Input: part model. Units: mm. Frame: model coordinates. Face numbers are marked on the shaded views. A direction names the side the tool comes from. Coordinates: 2 decimals unless noted, no trailing zeros. Loops run counter-clockwise (first coordinate to the right, second up) from the corner with the lowest first, then second, coordinate; pieces in that order, holes last.
Item 1: Ray query, line 1 along Y through (x, z) = (0, 25); line 2 along Y through (x, z) = (0, 6.5); line 3 along Z through (x, y) = (-11, -6). Return the intervals inside material, ascending.
Item 2: Reachability of the marked faces 1, 2 and 3 from +Z, -Z, +X, -X, +Y, -Y: full face, straight path, thin tool, end or side. Return the list, or none.
Item 3: Section A-A on x = 0. Return loops of the section in (y, z), and give its area (3 significant figures).
Item 4: Section D-D on z = 20. Return loops of the section in (x, y), and give its area (3 significant figures).
Item 5: Pull-direction query (X, two-part tool) for the marked faces 4, 5 and 6; classes: released by +X, released by -X, zero draft, split by the parting line, or undercut.
Item 6: Section B-B on z = 7. Return loops of the section in (x, y).
Item 7: Section C-C on y = -21.5. Return loops of the section in (x, z).
Item 8: Contact query for flat-ended pins moving along their axis: P1, Ø4, axis at x = 28, z = 24, coming from the -Y side; P2, Ø1, axis at y = 32.5, z = 29.5, coming from the +X side; P3, Ø5.5, axis at x = 23.5, z = 5, coming from the -Y side; P4, Ø9, axis at x = 0, y = 0, coming from the +Z side. Output: stop coordinate, or through.
```python
from build123d import *

# Parameters (mm, degrees)
F0_R     = 39.624
F0_R_2   = 5.500002
F1_DEPTH = 12.7
F2_R     = 69.469
F2_R_2   = 39.624
F3_DEPTH = 21.7805
F5_DEPTH = 45.212


with BuildPart() as f1:
    # F0 (on Top) → F1 (new body)
    with BuildSketch(Plane.XY):
        Circle(F0_R)
        Circle(F0_R_2, mode=Mode.SUBTRACT)
    extrude(amount=F1_DEPTH)

    # F2 (on face) → F3 (join, symmetric)
    with BuildSketch(Plane.XY.offset(12.7)):
        Circle(F2_R)
        Circle(F2_R_2, mode=Mode.SUBTRACT)
    extrude(amount=F3_DEPTH, both=True)

    # F4 (on face) → F5 (cut)
    with BuildSketch(Plane.XY.offset(12.7)):
        Polygon((21.139988, -4.44315), (26.270496, -4.44315), (28.83575, 0), (26.270496, 4.44315), (21.139988, 4.44315), (18.574734, 0), align=None)
    extrude(amount=-F5_DEPTH, mode=Mode.SUBTRACT)


solid = f1.part
```
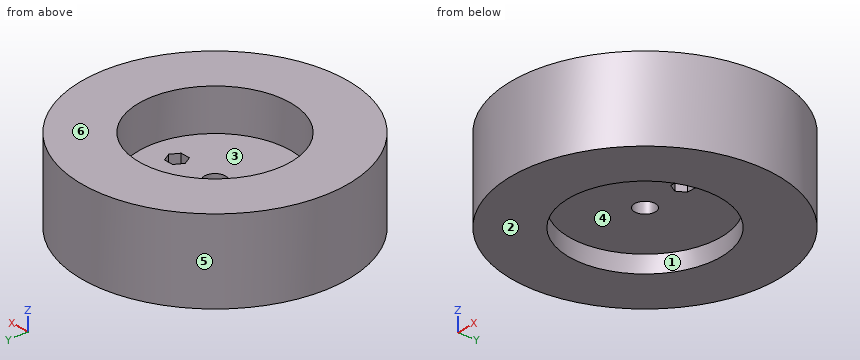
Results found:
1. line 1: y = -69.47 to -39.62, 39.62 to 69.47
1. line 2: y = -69.47 to -5.5, 5.5 to 69.47
1. line 3: z = 0 to 12.7
2. face 1: -Z
2. face 2: -Z, +X, -X, +Y, -Y
2. face 3: +Z
3. outline: (-69.47, -9.08) - (-39.62, -9.08) - (-39.62, 0) - (-5.5, 0) - (-5.5, 12.7) - (-39.62, 12.7) - (-39.62, 34.48) - (-69.47, 34.48) - close; (5.5, 0) - (39.62, 0) - (39.62, -9.08) - (69.47, -9.08) - (69.47, 34.48) - (39.62, 34.48) - (39.62, 12.7) - (5.5, 12.7) - close
3. area: 3,470 mm2
4. outline: circle Ø138.94 at (0, 0); hole circle Ø79.25 at (0, 0)
4. area: 10,200 mm2
5. face 4: undercut
5. face 5: split by the parting line
5. face 6: zero draft
6. outline: circle Ø138.94 at (0, 0); hole circle Ø11 at (0, 0); hole (18.57, 0) - (21.14, -4.44) - (26.27, -4.44) - (28.84, 0) - (26.27, 4.44) - (21.14, 4.44) - close
7. outline: (-66.06, -9.08) - (-33.28, -9.08) - (-33.28, 0) - (33.28, 0) - (33.28, -9.08) - (66.06, -9.08) - (66.06, 34.48) - (33.28, 34.48) - (33.28, 12.7) - (-33.28, 12.7) - (-33.28, 34.48) - (-66.06, 34.48) - close
8. P1: stops at y = -64.42
8. P2: stops at x = 61.66
8. P3: stops at y = -66.3
8. P4: passes through
